Can you work these out from the drawing? Everything is in mm from the part's minimum corner. Give positions to 0.01 mm unless a question says otherwise; leave off trailing zeros. Order: outer loops, then holes, each group sorted by start corner. A loop starts at its lowest first (then second) coordinate and runs counter-clockwise, first axis right, second up. Notation, with made-up numbers: (0.25, 86.5) - (13.25, 86.5) arc R9 cw to (13.25, 96.5) - close; hole circle Ø7 at (59.5, 83). An arc over 180 degrees is marked (long way). Answer as a JSON object with one key per item and string values.
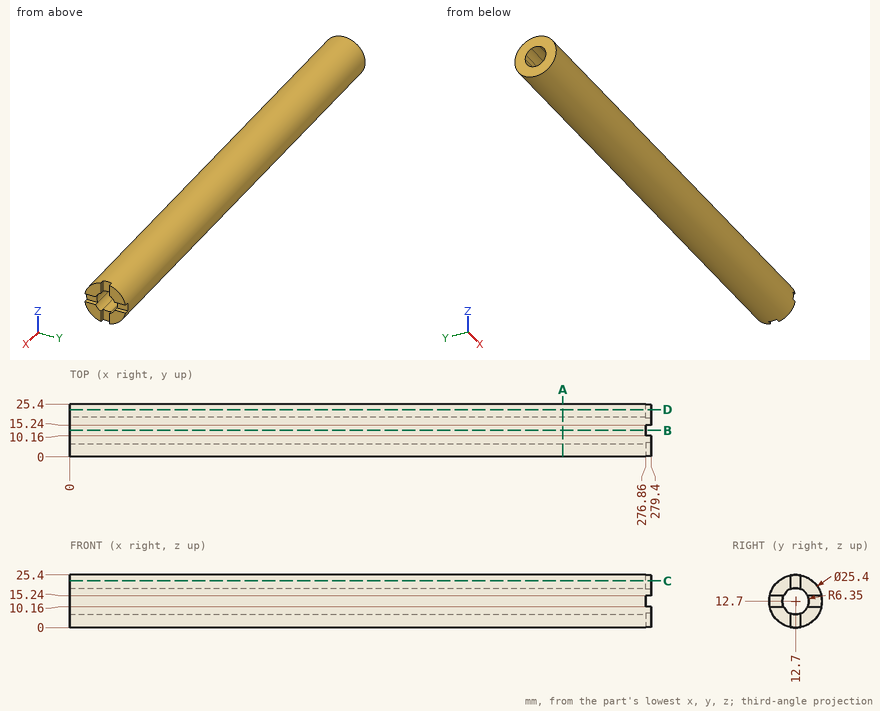
Q1. I need wall thicknesses on L1, parallel to Y at x = 29.5, z = 15.25; L2, parallel to Z at x = 33, y = 12.75; L3, parallel to Z at x = 129, y = 14.25. Which ranges of each line are inside material? Lowest first, please.
Recorded:
{"L1": "y = 0.26 to 6.88, 18.52 to 25.14", "L2": "z = 0 to 6.35, 19.05 to 25.4", "L3": "z = 0.09 to 6.54, 18.86 to 25.31"}
Q2. If we section it at D-D, the plane y = 22.75: Please give me the cut outline in (x, z).
Recorded:
{"outline": "(0, 4.94) - (279.4, 4.94) - (279.4, 10.16) - (276.86, 10.16) - (276.86, 15.24) - (279.4, 15.24) - (279.4, 20.46) - (0, 20.46) - close"}
Q3. I'm going to push flat-ended pins straight in: pin 1 Ø0.8 at (x, z) = (278, 3) entering from +Y; pin 2 Ø2.5 at (y, z) = (22.5, 12) entering from +X; pin 3 Ø3 at (x, z) = (278.5, 4.5) entering from -Y; pin 4 Ø4 at (x, y) = (67.5, 12) entering from +Z. Where does each tip first touch, or does it pass through?
Recorded:
{"pin 1": "stops at y = 21.35", "pin 2": "stops at x = 276.86", "pin 3": "stops at y = 1.91", "pin 4": "stops at z = 25.4"}
Q4. If we section it at B-B, the plane y = 12.7: Please give me the cut outline in (x, z), then the cut area to 3 significant figures.
Recorded:
{"outline": "(0, 0) - (276.86, 0) - (276.86, 6.35) - (0, 6.35) - close; (0, 19.05) - (276.86, 19.05) - (276.86, 25.4) - (0, 25.4) - close", "area": "3,520 mm^2"}
Q5. If we section it at A-A, the plane x = 237: Please give me the cut outline in (y, z), then the cut area to 3 significant figures.
Recorded:
{"outline": "circle Ø25.4 at (12.7, 12.7); hole (6.88, 10.16) arc R6.35 ccw to (10.16, 6.88) arc R6.35 ccw to (15.24, 6.88) arc R6.35 ccw to (18.52, 10.16) arc R6.35 ccw to (19.05, 12.7) arc R6.35 ccw to (18.52, 15.24) arc R6.35 ccw to (15.24, 18.52) arc R6.35 ccw to (10.16, 18.52) arc R6.35 ccw to (6.88, 15.24) arc R6.35 ccw to start", "area": "380 mm^2"}
Q6. If we section it at C-C, the plane z = 22.5: Please give me the cut outline in (x, y).
Recorded:
{"outline": "(0, 4.62) - (279.4, 4.62) - (279.4, 10.16) - (276.86, 10.16) - (276.86, 15.24) - (279.4, 15.24) - (279.4, 20.78) - (0, 20.78) - close"}
